Check sheet for the modelled part. Datum: model origin and axes. Units: mm. Give positions to 0.01 mm unless a question says otherwise; leave off trailing zeros. Loops run counter-clockwise (first coordinate to the right, second up) from the corner with the lowest first, then second, coordinate; pieces in that order, holes last.
```python
from build123d import *

# Parameters (mm, degrees)
BOSS_EXTRUDE1_DEPTH = 3.175
SKETCH2_R           = 4.8
CUT_EXTRUDE1_DEPTH  = 1


with BuildPart() as part:
    # Model → Boss-Extrude1 (new body)
    with BuildSketch(Plane.XY):
        with BuildLine():
            Line((175.500000042, 200), (125.500000042, 200))
            ThreePointArc((125.500000042, 200), (121.964466136, 198.535533906), (120.500000042, 195))
            Line((120.500000042, 195), (120.500000042, 177.5))
            ThreePointArc((120.500000042, 177.5), (119.035533948, 173.964466094), (115.500000042, 172.5))
            Line((115.500000042, 172.5), (-115.500000042, 172.5))
            ThreePointArc((-115.500000042, 172.5), (-119.035533948, 173.964466094), (-120.500000042, 177.5))
            Line((-120.500000042, 177.5), (-120.500000042, 195))
            ThreePointArc((-120.500000042, 195), (-121.964466136, 198.535533906), (-125.500000042, 200))
            Line((-125.500000042, 200), (-175.500000042, 200))
            ThreePointArc((-175.500000042, 200), (-179.035533948, 198.535533906), (-180.500000042, 195))
            Line((-180.500000042, 195), (-180.500000042, -195))
            ThreePointArc((-180.500000042, -195), (-179.035533948, -198.535533906), (-175.500000042, -200))
            Line((-175.500000042, -200), (-125.500000042, -200))
            ThreePointArc((-125.500000042, -200), (-121.964466136, -198.535533906), (-120.500000042, -195))
            Line((-120.500000042, -195), (-120.500000042, -177.5))
            ThreePointArc((-120.500000042, -177.5), (-119.035533948, -173.964466094), (-115.500000042, -172.5))
            Line((-115.500000042, -172.5), (115.500000042, -172.5))
            ThreePointArc((115.500000042, -172.5), (119.035533948, -173.964466094), (120.500000042, -177.5))
            Line((120.500000042, -177.5), (120.500000042, -195))
            ThreePointArc((120.500000042, -195), (121.964466136, -198.535533906), (125.500000042, -200))
            Line((125.500000042, -200), (175.500000042, -200))
            ThreePointArc((175.500000042, -200), (179.035533948, -198.535533906), (180.500000042, -195))
            Line((180.500000042, -195), (180.500000042, 195))
            ThreePointArc((180.500000042, 195), (179.035533948, 198.535533906), (175.500000042, 200))
        make_face()
        with BuildLine():
            Line((144.600753463, 187.910343452), (150.5, 187.910343452))
            ThreePointArc((150.5, 187.910343452), (153.089656548, 190.5), (150.5, 193.089656548))
            Line((150.5, 193.089656548), (144.600753463, 193.089656548))
            ThreePointArc((144.600753463, 193.089656548), (135.65, 190.5), (144.600753463, 187.910343452))
        make_face(mode=Mode.SUBTRACT)
        with BuildLine():
            Line((150.5, -187.910343452), (144.600753463, -187.910343452))
            ThreePointArc((144.600753463, -187.910343452), (135.65, -190.5), (144.600753463, -193.089656548))
            Line((144.600753463, -193.089656548), (150.5, -193.089656548))
            ThreePointArc((150.5, -193.089656548), (153.089656548, -190.5), (150.5, -187.910343452))
        make_face(mode=Mode.SUBTRACT)
        with BuildLine():
            Line((-150.5, -187.910343452), (-156.399246537, -187.910343452))
            ThreePointArc((-156.399246537, -187.910343452), (-165.35, -190.5), (-156.399246537, -193.089656548))
            Line((-156.399246537, -193.089656548), (-150.5, -193.089656548))
            ThreePointArc((-150.5, -193.089656548), (-147.910343452, -190.5), (-150.5, -187.910343452))
        make_face(mode=Mode.SUBTRACT)
        with BuildLine():
            Line((-150.5, 193.089656548), (-156.399246537, 193.089656548))
            ThreePointArc((-156.399246537, 193.089656548), (-165.35, 190.5), (-156.399246537, 187.910343452))
            Line((-156.399246537, 187.910343452), (-150.5, 187.910343452))
            ThreePointArc((-150.5, 187.910343452), (-147.910343452, 190.5), (-150.5, 193.089656548))
        make_face(mode=Mode.SUBTRACT)
    extrude(amount=BOSS_EXTRUDE1_DEPTH)

    # Sketch2 → Cut-Extrude1 (cut)
    with BuildSketch(Plane.XY.offset(3.175)):
        with Locations((-150.5, 190.5)):
            Circle(SKETCH2_R)
        with Locations((150.5, 190.5)):
            Circle(SKETCH2_R)
        with Locations((150.5, -190.5)):
            Circle(SKETCH2_R)
        with Locations((-150.5, -190.5)):
            Circle(SKETCH2_R)
    extrude(amount=-CUT_EXTRUDE1_DEPTH, mode=Mode.SUBTRACT)


solid = part.part
```
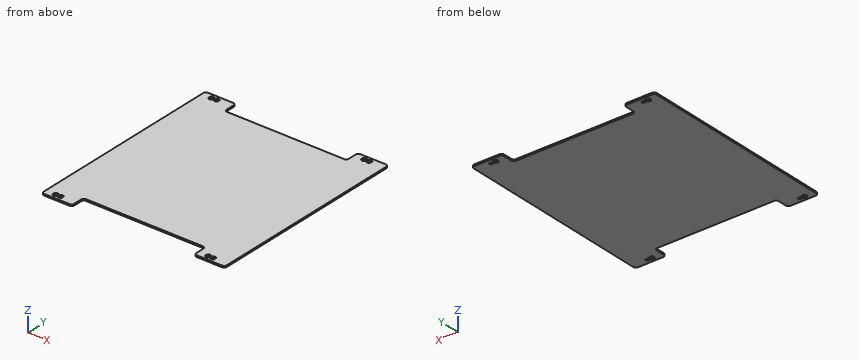
(1) Section check A-A on x = -90. Record the boundary of the cut face in (y, z) (3 decimals).
(2) Material ranges on line 1 (X direction, y = -190.5, z = 2.8); line 2 (X direction, y = -190.5, z = 1.55); line 3 (Y direction, x = 150.5, z = 2.5), recorded low to high.
(3) Gauge pin test, flat ends, axial feed: pin 1 Ø1 at (x, z) = (32, 1.5) entering from +Y; pin 2 Ø8.5 at (x, y) = (140.5, 190.5) entering from +Z; pin 3 Ø1 at (x, z) = (-23, 0.5) entering from -Y; pin 4 Ø4.5 at (x, y) = (-150.5, 192.5) entering from +Z (3 decimals). Record the tip position at first contact, or that the pin passes through.
Computed values:
1. outline: (-172.5, 0) - (172.5, 0) - (172.5, 3.175) - (-172.5, 3.175) - close
2. line 1: x = -180.5 to -165.35, -145.7 to -120.5, 120.5 to 135.65, 155.3 to 180.5
2. line 2: x = -180.5 to -165.35, -147.91 to -120.5, 120.5 to 135.65, 153.09 to 180.5
2. line 3: y = -200 to -195.3, -185.7 to 185.7, 195.3 to 200
3. pin 1: stops at y = 172.5
3. pin 2: passes through
3. pin 3: stops at y = -172.5
3. pin 4: stops at z = 2.175
